```python
from build123d import *

# Parameters (mm, degrees)
F1_DEPTH = 12
F2_R     = 1.1
F3_DEPTH = 12.001
F4_R     = 2


with BuildPart() as f1:
    # F0 (on Top) → F1 (new body)
    with BuildSketch(Plane.XY):
        Polygon((0, 17), (0, 0), (64.6, 0), (64.6, 58.6), (64.6, 64.6), (47.6, 64.6), (47.6, 58.6), (54.6, 58.6), (54.6, 10), (6, 10), (6, 17), align=None)
    extrude(amount=F1_DEPTH)

    # F2 (on Top) → F3 (cut, through all)
    with BuildSketch(Plane.XY):
        with Locations((6, 11.1)):
            Circle(F2_R)
        with Locations((53.5, 58.6)):
            Circle(F2_R)
    extrude(amount=F3_DEPTH, mode=Mode.SUBTRACT)

    # F4
    f4_edges = [f1.edges().sort_by_distance(p)[0] for p in [
        (0, 0, 6),
        (64.6, 0, 6),
        (32.3, 0, 0),
        (32.3, 0, 12),
        (0, 17, 6),
        (0, 8.5, 0),
        (0, 8.5, 12),
        (64.6, 32.3, 12),
        (64.6, 64.6, 6),
        (64.6, 32.3, 0),
        (47.6, 64.6, 6),
        (56.1, 64.6, 0),
        (56.1, 64.6, 12),
    ]]
    fillet(f4_edges, radius=F4_R)


solid = f1.part
```
Geometry: final body of the model. Coordinates: model frame, mm. A direction names the side the tool comes from. Coordinates: 2 decimals unless noted, no trailing zeros. Loops run counter-clockwise (first coordinate to the right, second up) from the corner with the lowest first, then second, coordinate; pieces in that order, holes last. Notation, with made-up numbers: (40, -9) -> (52, -9) arc R24 ccw to (52, 3) -> close; hole circle Ø1 at (66, 17.25). An arc over 180 degrees is marked (long way). Use a Markdown table: item, result. Add a question column.
(1) Section query C-C, the plane z = 4.5. Return loops of the section in (x, y), plus the area to 3 significant figures.
(2) Section query D-D, the plane x = 36. Return loops of the section in (y, z), plus the area to 3 significant figures.
(3) Pin query (flat end, axial travel): pin 1 Ø2 at (y, z) = (60, 4.5) entering from -X; pin 2 Ø3 at (x, z) = (14.5, 7) entering from +Y; pin 3 Ø2 at (x, z) = (4, 7.5) entering from +Y; pin 4 Ø10 at (x, y) = (50, 38.5) entering from -Z. Return the tip coordinate at first contact, or that it passes through.
(4) Mould query, pull axis X, two halves, no side actions, for faces 1 (the cylindrical face through (53.5, 59.7, 5.9)), 2 (the cylindrical face through (0.57, 9.4, 0.6)), 3 (the flat face through (55, 23, 0)). Classes: pulls with the +X half, pulls with the -X half, needs draft (parallel to the pull), parting line crosses it, or undercut.
(5) Section query B-B, the plane x = 53.5. Return loops of the section in (y, z).
(6) Section query A-A, the plane y = 11.1. Return loops of the section in (x, z).
(7) Line query: line 1 along Y through (x, z) = (50, 8.5); line 2 along X through (y, z) = (29, 7.5); line 3 along Y through (x, z) = (45, 4.5). Output: solid intervals per line, ascending.
(8) Access query for faces 4 (the cylindrical face through (4.9, 11.1, 5.9)), 5 (the flat face through (50, 58.6, 6)), 6 (the cylindrical face through (64, 32.72, 11.43)), 7 (the flat face through (0, 9, 6)), 8 (the flat face through (4, 17, 6)). Directions: +Z, -Z, +X, -X, +Y, -Y. A direction counts if a zero-diameter tool reaches every point of the face in a straight line with its end or side. Return the directions, or none.
Answer:
| question | item | result |
|---|---|---|
| 1 | outline | (0, 2) arc R2 ccw to (2, 0) -> (62.6, 0) arc R2 ccw to (64.6, 2) -> (64.6, 62.6) arc R2 ccw to (62.6, 64.6) -> (49.6, 64.6) arc R2 ccw to (47.6, 62.6) -> (47.6, 58.6) -> (52.4, 58.6) arc R1.1 cw to (54.6, 58.6) -> (54.6, 10) -> (6, 10) arc R1.1 cw to (6, 12.2) -> (6, 17) -> (2, 17) arc R2 ccw to (0, 15) -> close |
| 1 | area | 1,270 mm^2 |
| 2 | outline | (0, 2) arc R2 ccw to (2, 0) -> (10, 0) -> (10, 12) -> (2, 12) arc R2 ccw to (0, 10) -> close |
| 2 | area | 118 mm^2 |
| 3 | pin 1 | stops at x = 47.6 |
| 3 | pin 2 | stops at y = 10 |
| 3 | pin 3 | stops at y = 17 |
| 3 | pin 4 | stops at z = 0 |
| 4 | face 1 | undercut |
| 4 | face 2 | pulls with the -X half |
| 4 | face 3 | needs draft |
| 5 | outline | (0, 2) arc R2 ccw to (2, 0) -> (10, 0) -> (10, 12) -> (2, 12) arc R2 ccw to (0, 10) -> close; (59.7, 0) -> (62.6, 0) arc R2 ccw to (64.6, 2) -> (64.6, 10) arc R2 ccw to (62.6, 12) -> (59.7, 12) -> close |
| 6 | outline | (0, 2) arc R2 ccw to (2, 0) -> (4.9, 0) -> (4.9, 12) -> (2, 12) arc R2 ccw to (0, 10) -> close; (54.6, 0) -> (62.6, 0) arc R2 ccw to (64.6, 2) -> (64.6, 10) arc R2 ccw to (62.6, 12) -> (54.6, 12) -> close |
| 7 | line 1 | y = 0 to 10, 58.6 to 64.6 |
| 7 | line 2 | x = 54.6 to 64.6 |
| 7 | line 3 | y = 0 to 10 |
| 8 | face 4 | +Z, -Z |
| 8 | face 5 | +Z, -Z, -X |
| 8 | face 6 | +Z, +X, +Y, -Y |
| 8 | face 7 | +Z, -Z, -X, +Y, -Y |
| 8 | face 8 | +Z, -Z, -X, +Y |
